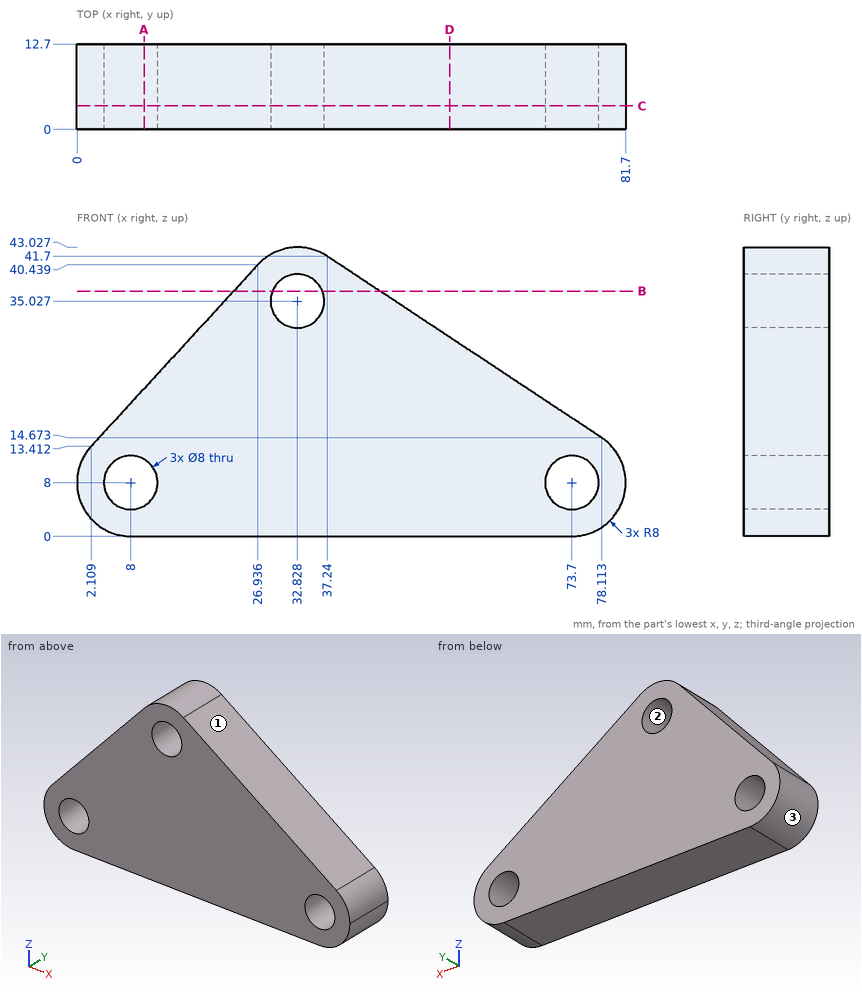
Part print with two shaded views. Sizes in mm from the minimum x, y, z corner. Coordinates: 2 decimals unless noted, no trailing zeros. Order: outer loops, then holes, each group sorted by start corner. A loop starts at its lowest first (then second) coordinate and runs counter-clockwise, first axis right, second up.
(1) Pin check, flat tips, straight feed: pin 1 Ø2 at (y, z) = (7.5, 9.5) entering from -X; pin 2 Ø3 at (y, z) = (2, 23.5) entering from +X; pin 3 Ø2 at (x, y) = (46, 11) entering from +Z. Stop position of each tip, or through.
Solution:
pin 1: stops at x = 0.02
pin 2: stops at x = 67.03
pin 3: stops at z = 36.57
(2) Drill centre lines: L1, parallel to Z at x = 8, y = 9.25 (1 decimal); L2, parallel to X at y = 4.25, z = 8.5 (1 decimal); L3, parallel to Z at x = 73.7, y = 9. Where is each one in solid material? Low to high.
Solution:
L1: z = 0 to 4, 12 to 19.8
L2: x = 0 to 4, 12 to 69.7, 77.7 to 81.7
L3: z = 0 to 4, 12 to 17.59
(3) Saw through at A-A, the plane x = 10. Write the cut outline in (y, z) (1 decimal).
Solution:
outline: (0, 0) - (12.7, 0) - (12.7, 4.5) - (0, 4.5) - close; (0, 11.5) - (12.7, 11.5) - (12.7, 22) - (0, 22) - close
(4) Saw through at B-B, the plane z = 36.5. Write the cut outline in (x, y) (1 decimal), and give its area (3 significant figures).
Solution:
outline: (23.3, 0) - (29.1, 0) - (29.1, 12.7) - (23.3, 12.7) - close; (36.5, 0) - (45.1, 0) - (45.1, 12.7) - (36.5, 12.7) - close
area: 182 mm2
(5) Mould opens along Z. For the marked faces 1, 2 and 3 say: released by +Z, released by -Z, zero draft, split by the parting line, or undercut.
Solution:
face 1: released by +Z
face 2: undercut
face 3: split by the parting line
(6) Saw through at D-D, the plane x = 55.5. Write the cut outline in (y, z) (1 decimal).
Solution:
outline: (0, 0) - (12.7, 0) - (12.7, 29.6) - (0, 29.6) - close
(7) Saw through at C-C, the plane y = 3.5. Write the cut outline in (x, z), and give its area (3 significant figures).
Solution:
outline: (2.11, 13.41) arc R8 ccw to (8, 0) - (73.7, 0) arc R8 ccw to (78.11, 14.67) - (37.24, 41.7) arc R8 ccw to (26.94, 40.44) - close; hole circle Ø8 at (8, 8); hole circle Ø8 at (32.83, 35.03); hole circle Ø8 at (73.7, 8)
area: 2,150 mm2
